Autodesk Inventor part; units mm, degrees
ref_plane "YZ Plane" through (0, 0, 0) normal (1, 0, 0) x (0, 1, 0)
ref_plane "XZ Plane" through (0, 0, 0) normal (0, 1, 0) x (-1, 0, 0)
ref_plane "XY Plane" through (0, 0, 0) normal (0, 0, 1) x (1, 0, 0)
ref_plane "Work Plane1" through (0, 0, 0) normal (0, 0, 1) x (1, 0, 0)
sketch "Sketch1" plane through (0, 0, 0) normal (0, 0, 1) x (1, 0, 0)
  arc A0 (-18.155, 30) -> (-18.155, 0) centre (0, 15) ccw construction
  line L0 (-18.155, 0) -> (-3.4871, 0) construction
  line L1 (-18.155, 30) -> (-3.4871, 30) construction
  circle A1 centre (0, 15) radius 15.4 construction
  arc A2 (-6.5238, 29.25) -> (-6.5238, 0.75) centre (0, 15) ccw construction
  line L2 (-6.5238, 0.75) -> (-17.7982, 0.75) construction
  arc A3 (-17.7982, 29.25) -> (-17.7982, 0.75) centre (0, 15) ccw construction
  line L3 (-17.7982, 29.25) -> (-6.5238, 29.25) construction
  circle A4 centre (0, 15) radius 12.775 construction
  line L4 (-6.5238, 29.25) -> (0, 29.25) construction
  line L5 (-6.5238, 0.75) -> (0, 0.75) construction
  arc A5 (0, 0.75) -> (0, 29.25) centre (0, 15) ccw construction
  line L6 (-42.0841, 29.25) -> (-42.0841, 0.75)
  line L7 (-42.0841, 0.75) -> (0, 0.75)
  line L8 (-42.0841, 29.25) -> (0, 29.25)
  circle A6 centre (0, 15) radius 11.5
  arc A7 (0, 0.75) -> (0, 29.25) centre (0, 15) ccw
  arc A8 (-3.4871, 0) -> (3.4871, 0) centre (0, 15) ccw
  line L9 (3.4871, 0) -> (18, 0)
  line L10 (18, 0) -> (18, 30)
  line L11 (3.4871, 30) -> (18, 30)
  arc A9 (3.4871, 30) -> (-3.4871, 30) centre (0, 15) ccw
  line L12 (-7.3927, 28.5095) -> (7.3927, 28.5095)
  arc A10 (7.3927, 1.4905) -> (7.3927, 28.5095) centre (0, 15) ccw
  line L13 (7.3927, 1.4905) -> (-7.3927, 1.4905)
  arc A11 (-7.3927, 28.5095) -> (-7.3927, 1.4905) centre (0, 15) ccw
  point P0 (0, 0)
  dimension "d0" = 0.75
  dimension "d1" = 25.55
  dimension "d2" = 23
extrude "Extrusion1" add sketch "Sketch1" along normal blind 1 contours L8 A7 L12 A11 L13 L7 L6 | A7 L13 A11 L12
sketch "Sketch2" plane through (0, 0, 1) normal (0, 0, 1) x (1, 0, 0)
  circle A0 centre (0, 15) radius 11.5
  line L0 (0, 29.25) -> (-42.0841, 29.25)
  line L1 (-42.0841, 29.25) -> (-42.0841, 0.75)
  line L2 (-42.0841, 0.75) -> (0, 0.75)
  arc A1 (0, 0.75) -> (0, 29.25) centre (0, 15) ccw
  circle A2 centre (0, 15) radius 12.775
  point P0 (0, 0)
  dimension "d5" = 25.55
extrude "Extrusion2" add sketch "Sketch2" along normal blind 6.25 contours A1 L2 L1 L0
properties part number "10_Filteslide_25mm"
Geometry check sheet. Reference: the model listing, model coordinates, mm. A direction names the side the tool comes from. Give positions to 0.01 mm unless a question says otherwise; leave off trailing zeros. Order: outer loops, then holes, each group sorted by start corner. A loop starts at its lowest first (then second) coordinate and runs counter-clockwise, first axis right, second up.
1. Sectioned sample at C-C (x = 2). Record the boundary of the cut face in (y, z), then the cut area to 3 significant figures.
Completed:
outline: (0.89, 0) - (3.68, 0) - (3.68, 1) - (2.38, 1) - (2.38, 7.25) - (0.89, 7.25) - close; (26.32, 0) - (29.11, 0) - (29.11, 7.25) - (27.62, 7.25) - (27.62, 1) - (26.32, 1) - close
area: 24.2 mm2
2. Draft check along Y on faces 1 (the face through (14.247, 15.313, 3.574)), 2 (the face through (-21, 0.75, 4)), 3 (the face through (-1.5, 3.6, 0.5)), 4 (the face through (-42.084, 15, 4)). Enter one of: pulls with the +Y half, pulls with the -Y half, needs draft (parallel to the pull), parting line crosses it, or undercut.
Completed:
face 1: parting line crosses it
face 2: pulls with the -Y half
face 3: undercut
face 4: needs draft
3. Depth check by flat-ended pin: pin 1 (3 mm diameter, centred on y = 8.5, z = 3.5, fed in from +X). Enter the tip coordinate at first touch or a pass-through.
Completed:
pin 1: stops at x = 13.34
4. Access from +Z, -Z, +X, -X, +Y, -Y to the whole of each face (thin tool, end or side, straight path). Record for faces 5 (the face through (-21, 15, 7.25)), 6 (the face through (-1.663, 2.334, 4.081)).
Completed:
face 5: +Z, +X, -X, +Y, -Y
face 6: +Z
5. Sectioned sample at A-A (y = 15). Record the boundary of the cut face in (x, z) (3 decimals), then the cut area to 3 significant figures.
Completed:
outline: (-42.084, 0) - (-11.5, 0) - (-11.5, 1) - (-12.775, 1) - (-12.775, 7.25) - (-42.084, 7.25) - close; (11.5, 0) - (14.25, 0) - (14.25, 7.25) - (12.775, 7.25) - (12.775, 1) - (11.5, 1) - close
area: 226 mm2
6. Scan lines: line 1 (Y direction, x = 0, z = 3.5) (3 decimals); line 2 (Y direction, x = 0, z = 0.5); line 3 (X direction, y = 17, z = 1.5). Record each from-to range of solid material in increasing order.
Completed:
line 1: y = 0.75 to 2.225, 27.775 to 29.25
line 2: y = 0.75 to 3.5, 26.5 to 29.25
line 3: x = -42.08 to -12.62, 12.62 to 14.11
7. Sectioned sample at B-B (z = 6). Record the boundary of the cut face in (x, y) (3 decimals).
Completed:
outline: (-42.084, 0.75) - (0, 0.75) arc R14.25 ccw to (0, 29.25) - (-42.084, 29.25) - close; hole circle Ø25.55 at (0, 15)
